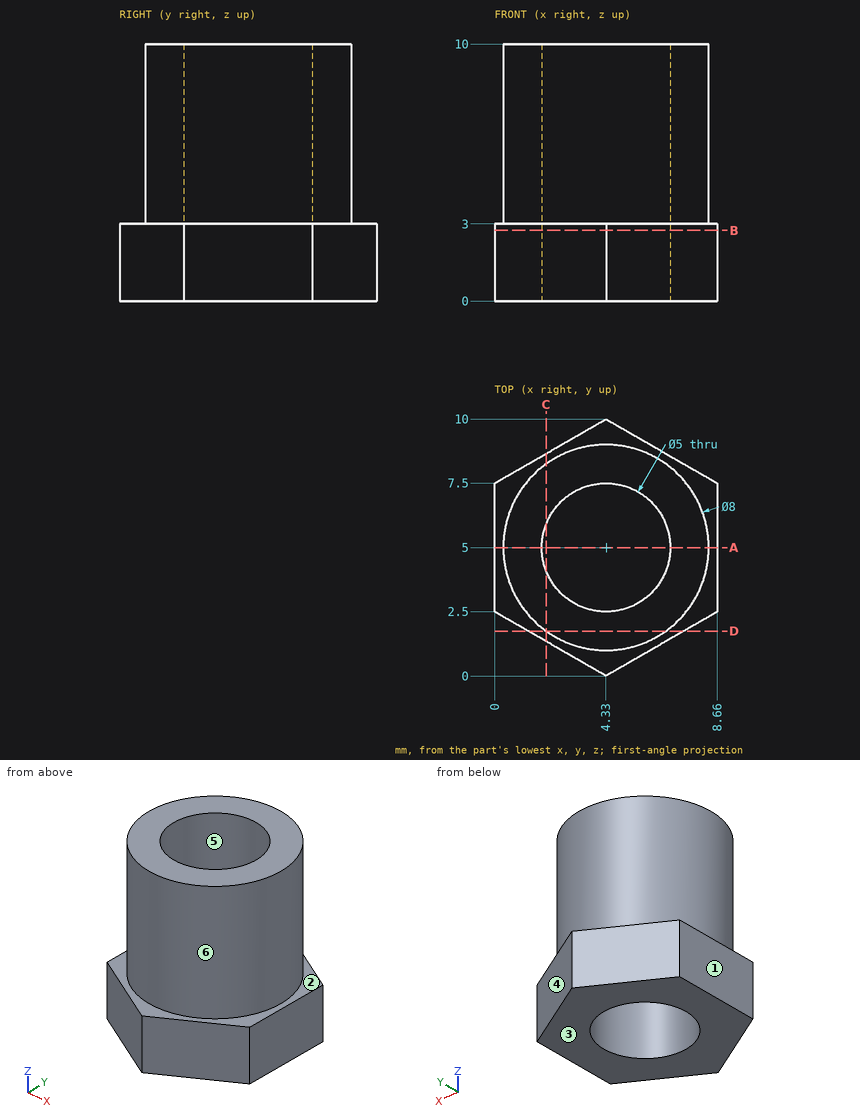
Verification items for this drawing (mm, ordinates from the low corner). A direction names the side the tool comes from. Coordinates: 2 decimals unless noted, no trailing zeros. Order: outer loops, then holes, each group sorted by start corner. A loop starts at its lowest first (then second) coordinate and runs counter-clockwise, first axis right, second up. Notation, with made-up numbers: (55, 16.5) - (62, 16.5) arc R26 ccw to (62, 41.5) - close; hole circle Ø8 at (69.5, 42.25). An arc over 180 degrees is marked (long way). Answer in a Markdown table with one row per item. Add a question column.
1. Draft check along X on the marked faces 3, 4, 5 and 6. Enter one of: +X half, -X half, draft (parallel to the pull), parting line (faces both ways), or undercut.
2. Section check D-D (y = 1.75). Enter the section's corners in (x, z).
3. Section check C-C (x = 2). Enter the section's corners in (y, z) (1 decimal).
4. Section check B-B (z = 2.75). Enter the section's corners in (x, y).
5. Access from +Z, -Z, +X, -X, +Y, -Y to the whole of each face (thin tool, end or side, straight path). Record for the marked faces 1 and 2.
6. Gauge pin test, flat ends, axial feed: pin 1 Ø2 at (x, z) = (7.5, 7) entering from +Y; pin 2 Ø1 at (y, z) = (6.5, 7.5) entering from +X; pin 3 Ø3 at (x, y) = (2, 2.5) entering from -Z; pin 4 Ø5 at (x, z) = (8, 3) entering from -Y (1 decimal). Record the tip position at first contact, or that the pin passes through.
7. Section check A-A (y = 5). Enter the section's corners in (x, z).
8. Material ranges on L1, parallel to X at y = 5, z = 2.75; L2, parallel to X at y = 6.5, z = 1.5; L3, parallel to Y at x = 3.75, z = 5, recorded low to high. Write a range as [from, to].
Data:
| question | item | result |
|---|---|---|
| 1 | face 3 | draft |
| 1 | face 4 | +X half |
| 1 | face 5 | undercut |
| 1 | face 6 | parting line |
| 2 | outline | (1.3, 0) - (7.36, 0) - (7.36, 3) - (6.66, 3) - (6.66, 10) - (2, 10) - (2, 3) - (1.3, 3) - close |
| 3 | outline | (1.3, 0) - (4.1, 0) - (4.1, 10) - (1.7, 10) - (1.7, 3) - (1.3, 3) - close; (5.9, 0) - (8.7, 0) - (8.7, 3) - (8.3, 3) - (8.3, 10) - (5.9, 10) - close |
| 4 | outline | (0, 2.5) - (4.33, 0) - (8.66, 2.5) - (8.66, 7.5) - (4.33, 10) - (0, 7.5) - close; hole circle Ø5 at (4.33, 5) |
| 5 | face 1 | +Z, -Z, -X, +Y, -Y |
| 5 | face 2 | +Z |
| 6 | pin 1 | stops at y = 8.36 |
| 6 | pin 2 | stops at x = 8.2 |
| 6 | pin 3 | stops at z = 0 |
| 6 | pin 4 | stops at y = 0.7 |
| 7 | outline | (0, 0) - (1.83, 0) - (1.83, 10) - (0.33, 10) - (0.33, 3) - (0, 3) - close; (6.83, 0) - (8.66, 0) - (8.66, 3) - (8.33, 3) - (8.33, 10) - (6.83, 10) - close |
| 8 | L1 | x = [0, 1.83], [6.83, 8.66] |
| 8 | L2 | x = [0, 2.33], [6.33, 8.66] |
| 8 | L3 | y = [1.04, 2.57], [7.43, 8.96] |
